```python
from build123d import *

# Parameters (mm, degrees)
F1_DEPTH = 6.35


with BuildPart() as f1:
    # F0 (on Top) → F1 (new body)
    with BuildSketch(Plane.XY):
        with BuildLine():
            ThreePointArc((17.789634, 31.521532), (0, 27.491055), (-17.789634, 31.521532))
            ThreePointArc((-17.789634, 31.521532), (-31.345789, 18.0975), (-36.193264, -0.354491))
            ThreePointArc((-36.193264, -0.354491), (-23.807952, -13.745528), (-18.40363, -31.167041))
            ThreePointArc((-18.40363, -31.167041), (0, -36.195), (18.40363, -31.167041))
            ThreePointArc((18.40363, -31.167041), (23.807952, -13.745528), (36.193264, -0.354491))
            ThreePointArc((36.193264, -0.354491), (31.345789, 18.0975), (17.789634, 31.521532))
        make_face()
        with BuildLine():
            ThreePointArc((-1.904548, -33.092239), (-8.919605, -31.924352), (-15.524087, -29.286965))
            ThreePointArc((-15.524087, -29.286965), (-17.182659, -21.372657), (-20.251486, -13.891384))
            Line((-20.251486, -13.891384), (-4.753306, -4.943505))
            ThreePointArc((-4.753306, -4.943505), (-3.429, -5.939202), (-1.904548, -6.588237))
            Line((-1.904548, -6.588237), (-1.904548, -33.092239))
        make_face(mode=Mode.SUBTRACT)
        with BuildLine():
            ThreePointArc((15.524087, -29.286965), (8.920041, -31.92423), (1.905452, -33.092187))
            Line((1.905452, -33.092187), (1.905452, -6.587975))
            ThreePointArc((1.905452, -6.587975), (3.429, -5.939202), (4.752628, -4.944157))
            Line((4.752628, -4.944157), (20.251068, -13.892186))
            ThreePointArc((20.251068, -13.892186), (17.182526, -21.373089), (15.524087, -29.286965))
        make_face(mode=Mode.SUBTRACT)
        with BuildLine():
            Line((-29.611197, 14.896328), (-6.657967, 1.644275))
            ThreePointArc((-6.657967, 1.644275), (-6.858, 0.000235), (-6.65808, -1.643818))
            Line((-6.65808, -1.643818), (-22.15652, -10.591846))
            ThreePointArc((-22.15652, -10.591846), (-27.100901, -4.19396), (-33.125299, 1.199229))
            ThreePointArc((-33.125299, 1.199229), (-32.107159, 8.237352), (-29.611197, 14.896328))
        make_face(mode=Mode.SUBTRACT)
        with BuildLine():
            Line((-4.752967, 4.943831), (-27.706197, 18.195885))
            ThreePointArc((-27.706197, 18.195885), (-23.187335, 23.686939), (-17.601212, 28.087736))
            ThreePointArc((-17.601212, 28.087736), (-9.917934, 25.566948), (-1.904548, 24.483993))
            Line((-1.904548, 24.483993), (-1.904548, 6.588237))
            ThreePointArc((-1.904548, 6.588237), (-3.428796, 5.93932), (-4.752967, 4.943831))
        make_face(mode=Mode.SUBTRACT)
        with BuildLine():
            ThreePointArc((-3.81, 0), (0, 3.81), (3.81, 0))
            ThreePointArc((3.81, 0), (0, -3.81), (-3.81, 0))
        make_face(mode=Mode.SUBTRACT)
        with BuildLine():
            ThreePointArc((29.610627, 14.897462), (32.107001, 8.237967), (33.125299, 1.199229))
            ThreePointArc((33.125299, 1.199229), (27.100593, -4.194291), (22.156034, -10.59261))
            Line((22.156034, -10.59261), (6.657854, -1.644731))
            ThreePointArc((6.657854, -1.644731), (6.858, 0.000424), (6.657651, 1.645555))
            Line((6.657651, 1.645555), (29.610627, 14.897462))
        make_face(mode=Mode.SUBTRACT)
        with BuildLine():
            ThreePointArc((17.601212, 28.087736), (23.186882, 23.687383), (27.705501, 18.196946))
            Line((27.705501, 18.196946), (4.752016, 4.944745))
            ThreePointArc((4.752016, 4.944745), (3.428632, 5.939414), (1.905452, 6.587975))
            Line((1.905452, 6.587975), (1.905452, 24.484032))
            ThreePointArc((1.905452, 24.484032), (9.918375, 25.567049), (17.601212, 28.087736))
        make_face(mode=Mode.SUBTRACT)
    extrude(amount=F1_DEPTH)


solid = f1.part
```
Could you check a few things on this model? Use its own coordinates, in mm. A direction names the side the tool comes from. Give positions to 0.01 mm unless a question says otherwise; leave off trailing zeros. Loops run counter-clockwise (first coordinate to the right, second up) from the corner with the lowest first, then second, coordinate; pieces in that order, holes last. Notation, with made-up numbers: (28.5, 7.5) - (33.5, 7.5) arc R26 ccw to (33.5, 26.5) - close; hole circle Ø1 at (33, -30). An arc over 180 degrees is marked (long way). Use one line per item in the form item = value.
1. Thinking about a two-plate mould opening in X: for faces 1 (the face through (-31.21, 18.33, 3.13)), 2 (the face through (-12.61, -9.48, 3.13)), 3 (the face through (0, -5, 6.35)), 4 (the face through (-0.27, -36.194, 3.131)), which applies, released by +X, released by -X, zero draft, split by the parting line, or undercut?
Response values:
face_1 = released by -X
face_2 = undercut
face_3 = zero draft
face_4 = split by the parting line
2. I want a section at B-B (y = -24). Please give me the cut outline in (x, z), and give its area (3 significant figures).
Response values:
outline = (-19.61, 0) - (-16.46, 0) - (-16.46, 6.35) - (-19.61, 6.35) - close; (-1.9, 0) - (1.91, 0) - (1.91, 6.35) - (-1.9, 6.35) - close; (16.46, 0) - (19.61, 0) - (19.61, 6.35) - (16.46, 6.35) - close
area = 64.1 mm²
3. I want a section at C-C (x = 24.5). Please give me the cut outline in (y, z), and give its area (3 significant figures).
Response values:
outline = (-12.59, 0) - (-7.26, 0) - (-7.26, 6.35) - (-12.59, 6.35) - close; (11.95, 0) - (16.35, 0) - (16.35, 6.35) - (11.95, 6.35) - close; (22.33, 0) - (26.64, 0) - (26.64, 6.35) - (22.33, 6.35) - close
area = 89.2 mm²
4. I need wall thicknesses on probe 1 along Y at (x, z) = (-21.5, 2); probe 2 along Y at (x, z) = (9.5, 2.25); probe 3 along X at (y, z) = (5.5, 3.5). Which ranges of each line are inside material? Lowest first, please.
Response values:
probe_1 = -18.4 to -10.21, 10.21 to 14.61, 25.23 to 29.12
probe_2 = -34.93 to -31.76, -7.69 to -3.29, 3.29 to 7.69, 25.47 to 28.6
probe_3 = -35.77 to -32.69, -13.34 to -5.72, -4.1 to 4.1, 5.71 to 13.33, 32.69 to 35.77
5. I want a section at A-A (x = 0). Please give me the cut outline in (y, z) (3 decimals), and give its area (3 significant figures).
Response values:
outline = (-36.195, 0) - (-3.81, 0) - (-3.81, 6.35) - (-36.195, 6.35) - close; (3.81, 0) - (27.491, 0) - (27.491, 6.35) - (3.81, 6.35) - close
area = 356 mm²
6. I'm going to push flat-ended pins straight in: pin 1 Ø1.9 at (y, z) = (13.5, 4.5) entering from +X; pin 2 Ø2 at (x, y) = (2, -22) entering from +Z; pin 3 Ø4.5 at (x, y) = (0, 0) entering from -Z; pin 4 Ø1.9 at (y, z) = (12.5, 3.5) entering from -X. Where does each tip first touch, or does it pass through?
Response values:
pin_1 = 33.95
pin_2 = 6.35
pin_3 = through
pin_4 = -34.3
7. On a 3-axis mill with a long thin cutter (end or side, diameter ignored), from which of +Z, -Z, +X, -X, +Y, -Y can I reach the whole of each face in a straight line? I mean faces 5 (the face through (0.26, 27.49, 3.13)), 6 (the face through (-8.82, -31.95, 3.13)). Say none if no direction works.
Response values:
face_5 = +Z, -Z, +Y
face_6 = +Z, -Z
8. I want a section at D-D (y = 11). Please give me the cut outline in (x, z).
Response values:
outline = (-34.48, 0) - (-31.27, 0) - (-31.27, 6.35) - (-34.48, 6.35) - close; (-22.86, 0) - (-15.24, 0) - (-15.24, 6.35) - (-22.86, 6.35) - close; (-1.9, 0) - (1.91, 0) - (1.91, 6.35) - (-1.9, 6.35) - close; (15.24, 0) - (22.86, 0) - (22.86, 6.35) - (15.24, 6.35) - close; (31.27, 0) - (34.48, 0) - (34.48, 6.35) - (31.27, 6.35) - close
